Verification items for the finished model (mm, model axes). A direction names the side the tool comes from. Coordinates: 2 decimals unless noted, no trailing zeros. Loops run counter-clockwise (first coordinate to the right, second up) from the corner with the lowest first, then second, coordinate; pieces in that order, holes last. Notation, with made-up numbers: (-26.5, 5) -> (13.5, 5) arc R25 cw to (13.5, 30) -> close; hole circle Ø1 at (-11.75, -0.5). An arc over 180 degrees is marked (long way). Use CSV: the item, a comma, the result in double quotes. Start each with the question number.
```python
from build123d import *

# Parameters (mm, degrees)
F0_R      = 11.85
F0_R_2    = 10.85
F1_DEPTH  = 9.5
F2_R      = 12.85
F2_R_2    = 10.85
F3_DEPTH  = 1
F4_R      = 2.35
F5_DEPTH  = 9.5
F6_R      = 1.15
F7_DEPTH  = 8
F8_SIZE   = 1
F10_SIZE  = 0.7
F12_DEPTH = 4.6
F13_COUNT = 6


with BuildPart() as f1:
    # F0 (on Top) → F1 (new body)
    with BuildSketch(Plane.XY):
        Circle(F0_R)
        Circle(F0_R_2, mode=Mode.SUBTRACT)
    extrude(amount=F1_DEPTH)

    # F2 (on face) → F3 (join)
    with BuildSketch(Plane(origin=(0, 0, 0), x_dir=(1, 0, 0), z_dir=(0, 0, -1))):
        Circle(F2_R)
        Circle(F2_R_2, mode=Mode.SUBTRACT)
    extrude(amount=F3_DEPTH)

    # F10
    f10_edges = [f1.edges().sort_by_distance(p)[0] for p in [
        (-10.85, 0, 9.5),
    ]]
    chamfer(f10_edges, length=F10_SIZE)



with BuildPart() as f5:
    # F4 (on face) → F5 (new body)
    with BuildSketch(Plane(origin=(0, 0, -1), x_dir=(1, 0, 0), z_dir=(0, 0, -1))):
        Circle(F4_R)
    extrude(amount=-F5_DEPTH)

    # F6 (on face) → F7 (cut)
    with BuildSketch(Plane(origin=(0, 0, -1), x_dir=(1, 0, 0), z_dir=(0, 0, -1))):
        Circle(F6_R)
    extrude(amount=-F7_DEPTH, mode=Mode.SUBTRACT)

    # F8
    f8_edges = [f5.edges().sort_by_distance(p)[0] for p in [
        (-2.35, 0, 8.5),
    ]]
    chamfer(f8_edges, length=F8_SIZE)


with BuildPart() as f1_1:
    add(f1.part)

    add(f5.part)  # F12 merges F5
    # F11 (on Top) → F12 (join)
    with BuildSketch(Plane.XY):
        with BuildLine():
            Line((-0.6, -2.2721135535), (-0.6, -10.8333974357))
            ThreePointArc((-0.6, -10.8333974357), (0, -10.85), (0.6, -10.8333974357))
            Line((0.6, -10.8333974357), (0.6, -2.2721135535))
            ThreePointArc((0.6, -2.2721135535), (0, -2.35), (-0.6, -2.2721135535))
        make_face()
    extrude(amount=F12_DEPTH)

    # F13: F1 ×6 about axis
    f13_axis = Axis((0, 0, 0), (0, 0, -1))


with BuildPart() as f1_2:
    add(f1_1.part)
    for i in range(1, F13_COUNT):
        add(f1_1.part.rotate(f13_axis, i * 360 / F13_COUNT))


solid = f1_2.part
```
1. Cross-section at A-A, the plane y = 0. Record the boundary of the cut face in (x, z).
2. Cross-section at B-B, the plane z = 3.75. Record the boundary of the cut face in (x, y), plus the area to 3 significant figures.
3. Release check for a two-part mould opening along X. For faces 5 (the flat face through (8.5, 8.5, 0)), 6 (the flat face through (-6.03, 2.79, 2.27)), 7 (the flat face through (5.43, 3.83, 2.27)) record: released by +X, released by -X, zero draft, split by the parting line, or undercut.
4. Scan lines: line 1 (Y direction, x = 0, z = 5); line 2 (Y direction, x = 0, z = 1.75); line 3 (X direction, y = 9.5, z = 1.25). Record each from-to range of solid material in increasing order.
5. Set-up check for faces 1 (the flat face through (-5.43, -3.83, 2.27)), 2 (the flat face through (-6, 3, 0)), 3 (the flat face through (-1, 1, -1)), 4 (the flat face through (0, 7, 4.6)): record each of +Z, -Z, +X, -X, +Y, -Y from which the full face is reachable in a straight line by a thin tool's end or side.
6. Cross-section at D-D, the plane x = -8.75. State how many separate pieces and enclosed holes the cut face has, plus the area to 3 significant figures.
7. Depth check by flat-ended pin: pin 1 (3.5 mm diameter, centred on x = 0, y = 0, fed in from +Z); pin 2 (3 mm diameter, centred on x = -2, z = 4, fed in from -Y); pin 3 (3.5 mm diameter, centred on y = 4.5, z = 2, fed in from -X). Enter the tip coordinate at first touch or a pass-through.
Solution:
1,outline,"(-12.85, -1) -> (-10.85, -1) -> (-10.85, 8.8) -> (-11.55, 9.5) -> (-11.85, 9.5) -> (-11.85, 0) -> (-12.85, 0) -> close; (-2.35, -1) -> (-1.15, -1) -> (-1.15, 7) -> (1.15, 7) -> (1.15, -1) -> (2.35, -1) -> (2.35, 7.5) -> (1.35, 8.5) -> (-1.35, 8.5) -> (-2.35, 7.5) -> close; (10.85, -1) -> (12.85, -1) -> (12.85, 0) -> (11.85, 0) -> (11.85, 9.5) -> (11.55, 9.5) -> (10.85, 8.8) -> close"
2,outline,"circle Ø23.7 at (0, 0); hole (-9.68, -4.9) -> (-2.27, -0.62) arc R2.35 cw to (-2.27, 0.62) -> (-9.68, 4.9) arc R10.85 ccw to start; hole (-9.08, -5.94) arc R10.85 ccw to (-0.6, -10.83) -> (-0.6, -2.27) arc R2.35 cw to (-1.67, -1.66) -> close; hole (-9.08, 5.94) -> (-1.67, 1.66) arc R2.35 cw to (-0.6, 2.27) -> (-0.6, 10.83) arc R10.85 ccw to start; hole circle Ø2.3 at (0, 0); hole (0.6, -10.83) arc R10.85 ccw to (9.08, -5.94) -> (1.67, -1.66) arc R2.35 cw to (0.6, -2.27) -> close; hole (0.6, 2.27) arc R2.35 cw to (1.67, 1.66) -> (9.08, 5.94) arc R10.85 ccw to (0.6, 10.83) -> close; hole (2.27, -0.62) -> (9.68, -4.9) arc R10.85 ccw to (9.68, 4.9) -> (2.27, 0.62) arc R2.35 cw to start"
2,area,"146 mm2"
3,face 5,"zero draft"
3,face 6,"undercut"
3,face 7,"undercut"
4,line 1,"y = -11.85 to -10.85, -2.35 to -1.15, 1.15 to 2.35, 10.85 to 11.85"
4,line 2,"y = -11.85 to -1.15, 1.15 to 11.85"
4,line 3,"x = -7.08 to -5.24, -0.6 to 0.6, 5.24 to 7.08"
5,face 1,"+Z, -Z"
5,face 2,"-Z"
5,face 3,"-Z, +X, -X, +Y, -Y"
5,face 4,"+Z"
6,separate pieces,"4"
6,enclosed holes,"0"
6,area,"47.9 mm2"
7,pin 1,"stops at z = 8.5"
7,pin 2,"stops at y = -11.84"
7,pin 3,"stops at x = -11.53"
